Model file for the job. Use its own axes, mm. Coordinates: 2 decimals unless noted, no trailing zeros. Order: outer loops, then holes, each group sorted by start corner. A loop starts at its lowest first (then second) coordinate and runs counter-clockwise, first axis right, second up. Notation, with made-up numbers: (86, 44) -> (97, 44) arc R10 cw to (97, 52) -> close; hole circle Ø10 at (53, -36.75). An arc over 180 degrees is marked (long way). Return JSON: item names as keys, results as strings. Group by question number.
1) Cut at A-A (z = -100). Write the cut outline in (x, y).
2) Cut at C-C (z = -40). Write the cut outline in (x, y), and give its area (3 significant figures).
3) Probe line 1 (Y direction, x = -1.45, z = -87.5); line 2 (Y direction, x = -1.1, z = -40); line 3 (Y direction, x = 0.85, z = -100). List the from-to ranges inside material, lowest first.
4) Flat gauge pin, fed straight in: pin 1 (3.5 mm diameter, centred on y = 12.5, z = -87.5, fed in from +X). Where does the tip first touch, or does it go through?
5) Cut at B-B (x = 0.1). State how many separate pieces and enclosed holes the cut face has, and give its area (3 significant figures).
from build123d import *

# Parameters (mm, degrees)
CROQUIS2_W                   = 235
CROQUIS2_H                   = 35
CROQUIS2_R                   = 4
CROQUIS2_R_2                 = 4.5
SALIENTE_EXTRUIR1_DEPTH      = 3
REDONDEO1_R                  = 5
TALADRO_DE_MARGEN_PARA_M41_D = 4.5
TALADRO_DE_MARGEN_PARA_M42_D = 4.5


with BuildPart() as part:
    # Croquis2 → Saliente-Extruir1 (new, symmetric)
    with BuildSketch(Plane(origin=(0, 0, 0), x_dir=(0, 0, -1), z_dir=(1, 0, 0))):
        Rectangle(CROQUIS2_W, CROQUIS2_H)
        with Locations((-100, 0)):
            Circle(CROQUIS2_R, mode=Mode.SUBTRACT)
        with Locations((100, 0)):
            Circle(CROQUIS2_R_2, mode=Mode.SUBTRACT)
    extrude(amount=SALIENTE_EXTRUIR1_DEPTH, both=True)

    # Redondeo1
    redondeo1_edges = [part.edges().sort_by_distance(p)[0] for p in [
        (0, 17.5, 117.5),
        (0, 17.5, -117.5),
        (0, -17.5, -117.5),
        (0, -17.5, 117.5),
    ]]
    fillet(redondeo1_edges, radius=REDONDEO1_R)

    # Taladro de margen para M41 (through all)
    with Locations(Plane(origin=(3, 0, 0), x_dir=(0, 0, -1), z_dir=(1, 0, 0))):
        with Locations((112.5, 12.5), (87.5, 12.5), (87.5, -12.5), (112.5, -12.5)):
            Hole(TALADRO_DE_MARGEN_PARA_M41_D / 2)

    # Taladro de margen para M42 (through all)
    with Locations(Plane(origin=(3, 0, 0), x_dir=(0, 0, -1), z_dir=(1, 0, 0))):
        with Locations((-40, 0), (40, 0)):
            Hole(TALADRO_DE_MARGEN_PARA_M42_D / 2)


solid = part.part
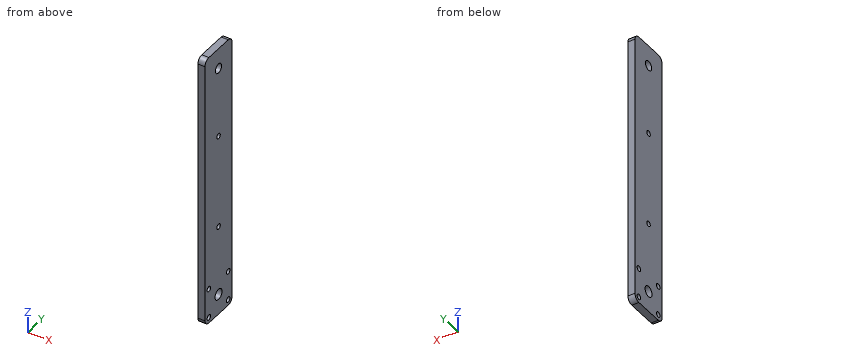
Answers below:
{
 "1": {"outline": "(-3, -17.5) -> (3, -17.5) -> (3, -4.5) -> (-3, -4.5) -> close; (-3, 4.5) -> (3, 4.5) -> (3, 17.5) -> (-3, 17.5) -> close"},
 "2": {"outline": "(-3, -17.5) -> (3, -17.5) -> (3, -2.25) -> (-3, -2.25) -> close; (-3, 2.25) -> (3, 2.25) -> (3, 17.5) -> (-3, 17.5) -> close", "area": "183 mm^2"},
 "3": {"line 1": "y = -17.5 to -14.75, -10.25 to 10.25, 14.75 to 17.5", "line 2": "y = -17.5 to -2.25, 2.25 to 17.5", "line 3": "y = -17.5 to -4.5, 4.5 to 17.5"},
 "4": {"pin 1": "passes through"},
 "5": {"separate pieces": "1", "enclosed holes": "8", "area": "7,990 mm^2"}
}
